Source: CAD feature listing. Evaluate the final solid. Frame: model axes, mm. Give positions to 0.01 mm unless a question says otherwise; leave off trailing zeros. Order: outer loops, then holes, each group sorted by start corner. A loop starts at its lowest first (then second) coordinate and runs counter-clockwise, first axis right, second up.
```python
from build123d import *

# Parameters (mm, degrees)
SKETCH1_R           = 2.1
SKETCH1_R_2         = 2.15
SKETCH1_R_3         = 2.2
SKETCH1_R_4         = 2
BOSS_EXTRUDE1_DEPTH = 8
FILLET1_R           = 4
CHAMFER1_SIZE       = 0.25


with BuildPart() as part:
    # Sketch1 → Boss-Extrude1 (new body)
    with BuildSketch(Plane(origin=(0, 0, 0), x_dir=(1, 0, 0), z_dir=(0, 1, 0))):
        Polygon((-6.92820323, 4), (0.690598923, -9.196152423), (11.309401077, -9.196152423), (18.92820323, 4), align=None)
        with Locations(Location((0, 0, 0), (0, 0, 270))):
            Circle(SKETCH1_R, mode=Mode.SUBTRACT)
        with Locations(Location((6, 0, 0), (0, 0, 270))):
            Circle(SKETCH1_R_2, mode=Mode.SUBTRACT)
        with Locations(Location((12, 0, 0), (0, 0, 270))):
            Circle(SKETCH1_R_3, mode=Mode.SUBTRACT)
        with Locations(Location((3, -5.196152423, 0), (0, 0, 270))):
            Circle(SKETCH1_R_4, mode=Mode.SUBTRACT)
        with Locations(Location((9, -5.196152423, 0), (0, 0, 270))):
            Circle(SKETCH1_R_4, mode=Mode.SUBTRACT)
    extrude(amount=BOSS_EXTRUDE1_DEPTH)

    # Fillet1
    fillet1_edges = [part.edges().sort_by_distance(p)[0] for p in [
        (18.92820323, 4, -4),
        (11.309401077, 4, 9.196152423),
        (0.690598923, 4, 9.196152423),
        (-6.92820323, 4, -4),
    ]]
    fillet(fillet1_edges, radius=FILLET1_R)

    # Chamfer1
    chamfer1_edges = [part.edges().sort_by_distance(p)[0] for p in [
        (0, 8, -2.1),
        (6, 8, -2.15),
        (12, 8, -2.2),
        (9, 8, 3.196152423),
        (3, 8, 3.196152423),
    ]]
    chamfer(chamfer1_edges, length=CHAMFER1_SIZE)


solid = part.part
```
1) Material intervals for L1, parallel to X at y = 3.5, z = 0; L2, parallel to Z at x = 1.75, y = 7.25; L3, parallel to Z at x = 4.5, y = 2.75, sorted ascending.
Report:
L1: x = -4 to -2.1, 2.1 to 3.85, 8.15 to 9.8, 14.2 to 16
L2: z = -4 to -1.16, 1.16 to 3.63, 6.76 to 9
L3: z = -4 to -1.54, 1.54 to 3.87, 6.52 to 9.2
2) Section query C-C, the plane y = 1.25. Return the cut outline in (x, z).
Report:
outline: (-3.46, 2) arc R4 ccw to (0, -4) - (12, -4) arc R4 ccw to (15.46, 2) - (12.46, 7.2) arc R4 ccw to (9, 9.2) - (3, 9.2) arc R4 ccw to (-0.46, 7.2) - close; hole circle Ø4.2 at (0, 0); hole circle Ø4 at (3, 5.2); hole circle Ø4.3 at (6, 0); hole circle Ø4 at (9, 5.2); hole circle Ø4.4 at (12, 0)
3) Section query D-D, the plane z = 4.25. Count the separate pieces of the cut face and the enclosed holes in it, and give its area (3 significant figures).
Report:
separate pieces: 3
enclosed holes: 0
area: 74.1 mm2
4) Pin query (flat end, axial travel): pin 1 (4 mm diameter, centred on x = 6, z = 0, fed in from +Y); pin 2 (1 mm diameter, centred on y = 5, z = -2.5, fed in from +X). Return the tip coordinate at first contact, or that it passes through.
Report:
pin 1: passes through
pin 2: stops at x = 15.46
5) Section query A-A, the plane x = 6. Return the cut outline in (y, z).
Report:
outline: (0, -4) - (8, -4) - (8, -2.4) - (7.75, -2.15) - (0, -2.15) - close; (0, 2.15) - (7.75, 2.15) - (8, 2.4) - (8, 9.2) - (0, 9.2) - close
6) Section query B-B, the plane z = 0. Return the cut outline in (x, y), and give its area (3 significant figures).
Report:
outline: (-4, 0) - (-2.1, 0) - (-2.1, 7.75) - (-2.35, 8) - (-4, 8) - close; (2.1, 0) - (3.85, 0) - (3.85, 7.75) - (3.6, 8) - (2.35, 8) - (2.1, 7.75) - close; (8.15, 0) - (9.8, 0) - (9.8, 7.75) - (9.55, 8) - (8.4, 8) - (8.15, 7.75) - close; (14.2, 0) - (16, 0) - (16, 8) - (14.45, 8) - (14.2, 7.75) - close
area: 56.6 mm2
7) Draft query along X for faces 1 (the cylindrical face through (-3.493, 4.056, -1.949)), 2 (the cylindrical face through (1.78, 3.82, 3.61)), 3 (the cylindrical face through (15.434, 4.056, -2.051)), 4 (the flat face through (6, 4, 9.196)). Return one class per face: +X half, -X half, draft (parallel to the pull), parting line (faces both ways), or undercut.
Report:
face 1: -X half
face 2: undercut
face 3: +X half
face 4: draft
